For this review, use the dimensioned drawing (mm, ordinates from the lowest corner) and the shaded views. A direction names the side the tool comes from. Round coordinates to 2 decimals unless told otherwise and drop trailing zeros. Write each loop counter-clockwise with the first axis right and the second up, starting at its lowest first coordinate (ties: lowest second). Pieces come first, ordered by that corner, then holes. Notation, with made-up numbers: M -25,15 L 29,15 A31 cw 29,44 Z; hole C 10,36.5 d1. An arc over 180 degrees is marked long. One line per question, with ' | ' between items. Start each with the question number.
Item 1: Draft analysis for pull direction Y (two halves, no side actions). For the marked faces 3, 4 and 5, state which applies: released by +Y, released by -Y, zero draft, split by the parting line, or undercut.
Item 2: Insertion check: pin 1 Ø12 at (x, y) = (12.5, 10) entering from -Z. The pin has a flat end and moves straight along its axis. Give the tip position at first contact, or say it passes through.
Item 3: For L1, parallel to X at y = 34, z = 1.5; L2, parallel to Y at x = 47.5, z = 4.75; L3, parallel to Z at x = 27, y = 32.5, list the stretches that pass through material, from the lowest coordinate up.
Item 4: Machinability: for the marked faces 1 and 2, which of the approach directions +Z, -Z, +X, -X, +Y, -Y give a long, thin tool a straight path to every point of the face, cutting with its end or side? Answer none if there is none.
Item 5: Add section A-A, the plane z = 1.75. State the section outline as (x, y) points, and give its area (3 significant figures).
Item 6: Add section C-C, the plane x = 28. State the section outline as (y, z) points.
Item 7: Add section B-B, the plane y = 11.5. State the section outline as (x, z) points, and give its area (3 significant figures).
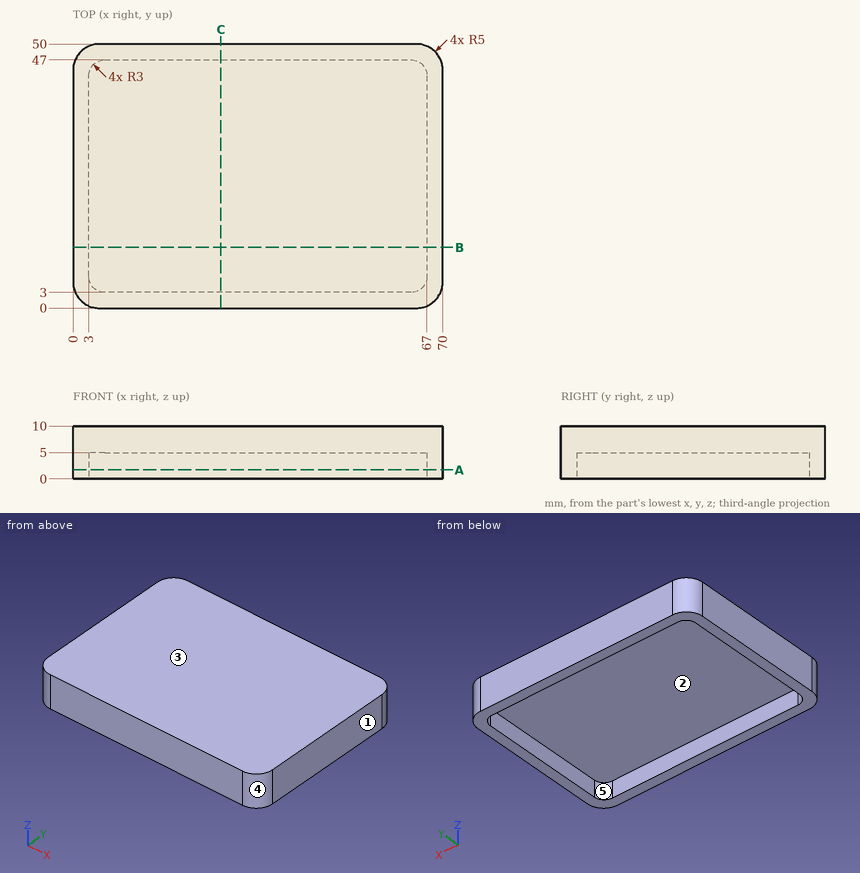
Computed values:
1) face 3: zero draft | face 4: released by -Y | face 5: undercut
2) pin 1: stops at z = 5
3) L1: x = 0 to 3, 67 to 70 | L2: y = 0 to 3, 47 to 50 | L3: z = 5 to 10
4) face 1: +Z, -Z, +X, +Y, -Y | face 2: -Z
5) outline: M 0,5 A5 ccw 5,0 L 65,0 A5 ccw 70,5 L 70,45 A5 ccw 65,50 L 5,50 A5 ccw 0,45 Z; hole M 3,6 A3 ccw 6,3 L 64,3 A3 ccw 67,6 L 67,44 A3 ccw 64,47 L 6,47 A3 ccw 3,44 Z | area: 670 mm^2
6) outline: M 0,0 L 3,0 L 3,5 L 47,5 L 47,0 L 50,0 L 50,10 L 0,10 Z
7) outline: M 0,0 L 3,0 L 3,5 L 67,5 L 67,0 L 70,0 L 70,10 L 0,10 Z | area: 380 mm^2
